```python
from build123d import *

# Parameters (mm, degrees)
FILLET1_SIZE              = 1.27
FILLET1_SIZE_2            = 12.7
SKETCH3_W                 = 3.175
SKETCH3_H                 = 3.175
CUT_EXTRUDE1_DEPTH        = 46.228
F_4_40_TAPPED_HOLE1_D     = 2.2606
F_4_40_TAPPED_HOLE1_DEPTH = 7.62
F_4_40_TAPPED_HOLE1_TIP   = 0.679152758
CIRPATTERN1_COUNT         = 4
BOSS_EXTRUDE1_DEPTH       = 41.402


# Read off the part's stored shape, not the designer's step: #6-32 Tapped Hole1
with BuildPart() as part:
    # Sketch2 → Revolve1 (revolve)
    with BuildSketch(Plane.XY, mode=Mode.PRIVATE) as revolve1_sk:
        Polygon((50.8, 0), (-115.824, 0), (-115.824, 4.7625), (-103.124, 4.7625), (-103.124, 38.862), (-10.16, 38.862), (-9.525, 38.227), (-9.525, 38.862), (0, 38.862), (0, 17.4498), (4.572, 17.4498), (4.572, 6.6675), (50.165, 6.6675), (50.8, 6.0325), align=None)
    revolve(revolve1_sk.sketch.rotate(Axis((88.99, 0, 0), (-1, 0, 0)), 90), axis=Axis((88.99, 0, 0), (-1, 0, 0)))

    # Fillet1
    # an asymmetric fillet: 12.7, 1.27 mm, written as the material it takes off along each edge
    with BuildSketch(Plane(origin=(-103.124, 0, 0), x_dir=(0, 0, -1), z_dir=(0, 1, 0))) as fillet1_piece_1:
        with BuildLine():
            Bezier((38.862 - FILLET1_SIZE, 0), (38.862, 0), (38.862, -FILLET1_SIZE_2), weights=[1, 0.707106781, 1])
            Line((38.862, -FILLET1_SIZE_2), (38.862, 0))
            Line((38.862, 0), (38.862 - FILLET1_SIZE, 0))
        make_face()
    revolve(axis=Axis((-103.124, 0, 0), (-1, 0, 0)), mode=Mode.SUBTRACT)

    # Sketch3 → Cut-Extrude1 (cut)
    with BuildSketch(Plane(origin=(50.8, 0, 0), x_dir=(0, 0, -1), z_dir=(1, 0, 0))):
        with Locations((0, 6.6675)):
            Rectangle(SKETCH3_W, SKETCH3_H)
    extrude(amount=-CUT_EXTRUDE1_DEPTH, mode=Mode.SUBTRACT)

    # Sketch8 → #8-32 Tapped Hole3 (revolve, cut)
    with BuildSketch(Plane(origin=(0, 0, -25), x_dir=(0, 0, -1), z_dir=(0, 1, 0))):
        Polygon((0, 0), (0, 11.705806461), (1.7272, 10.668), (1.7272, 0), align=None)
    f_8_32_tapped_hole3 = revolve(axis=Axis((6.35, 0, -25), (-1, 0, 0)), mode=Mode.SUBTRACT)

    # #6-32 Tapped Hole1 outline → #6-32 Tapped Hole1 (revolve, cut)
    with BuildSketch(Plane(origin=(0, 19.813624417, 28.296788218), x_dir=(0, 1, 0), z_dir=(0, 0, -1))):
        Polygon((1.35255, -93.726), (0, -92.91330597), (0, -103.124), (1.35255, -103.124), align=None)
    f_6_32_tapped_hole1 = revolve(axis=Axis((0, 19.813624417, 28.296788218), (1, 0, 0)), mode=Mode.SUBTRACT)

    # #4-40 Tapped Hole1
    with Locations(Plane.ZY.offset(103.124)):
        with Locations((-23, 0), (23, 0)):
            Hole(F_4_40_TAPPED_HOLE1_D / 2, depth=F_4_40_TAPPED_HOLE1_DEPTH)
            with Locations((0, 0, -(F_4_40_TAPPED_HOLE1_DEPTH + F_4_40_TAPPED_HOLE1_TIP / 2))):  # 118° drill point
                Cone(0, F_4_40_TAPPED_HOLE1_D / 2, F_4_40_TAPPED_HOLE1_TIP, mode=Mode.SUBTRACT)

    # CirPattern1: #8-32 Tapped Hole3, #6-32 Tapped Hole1 ×4 about axis
    cirpattern1_axis = Axis((0, 0, 0), (1, 0, 0))
    add([f_8_32_tapped_hole3.rotate(cirpattern1_axis, i * 360 / CIRPATTERN1_COUNT) for i in range(1, CIRPATTERN1_COUNT)], mode=Mode.SUBTRACT)
    add([f_6_32_tapped_hole1.rotate(cirpattern1_axis, i * 360 / CIRPATTERN1_COUNT) for i in range(1, CIRPATTERN1_COUNT)], mode=Mode.SUBTRACT)

    # Sketch12 → Boss-Extrude1 (add)
    with BuildSketch(Plane(origin=(0, 0, 0), x_dir=(1, 0, 0), z_dir=(0, 1, 0))):
        with BuildLine():
            Line((-92.964, -5.08), (-82.804, -5.08))
            ThreePointArc((-82.804, -5.08), (-77.724, 0), (-82.804, 5.08))
            Line((-82.804, 5.08), (-92.964, 5.08))
            Line((-92.964, 5.08), (-92.964, -5.08))
        make_face()
    extrude(amount=BOSS_EXTRUDE1_DEPTH)


solid = part.part
```
The model under review builds one solid part; all positions refer to its coordinate system, in mm. A direction names the side the tool comes from. Give positions to 0.01 mm unless a question says otherwise; leave off trailing zeros. Write each loop counter-clockwise with the first axis right and the second up, starting at its lowest first coordinate (ties: lowest second). Pieces come first, ordered by that corner, then holes.
(1) The part is to be moulded in two halves that separate along Y. For faces 4 (the cylindrical face through (27.688, -6.662, -0.271)), 5 (the flat face through (-115.824, 0, 0)), 6 (the conical face through (-11.526, -24.779, 0.203)), say which applies: released by +Y, released by -Y, zero draft, split by the parting line, or undercut.
(2) Consider section B-B, the plane x = -37. Give the boundary of the cut face in (y, z), and give its area (3 significant figures).
(3) For P1, Ø5.5, axis at y = 0, z = 25, coming from the +X side; P2, Ø12, axis at x = -44.5, y = 28, coming from the -Z side; P3, Ø3, axis at y = -25, z = 0, coming from the +X side, all flat-tipped, find the tip position at first contact; note any pin that passes through.
(4) Consider section C-C, the plane x = -88. Give the boundary of the cut face in (y, z).
(5) To check wall thickness, follow L1, parallel to X at y = -5.5, z = -9; L2, parallel to Z at x = -97.25, y = 0; L3, parallel to X at y = 31, z = 14. State the ranges of each line that lie inside material, in increasing order.
(6) Consider section A-A, the plane x = 28. Give the boundary of the cut face in (y, z) (1 decimal).
(7) Tool access review of faces 1 (the cylindrical face through (-109.39, 4.65, 1.03)), 2 (the cylindrical face through (-5.259, -23.274, 0.076)), 3 (the cylindrical face through (-77.725, 39.945, 0.112)): name each direction out of +Z, -Z, +X, -X, +Y, -Y from which nothing blocks a thin tool from reaching the whole face with its end or side.
Returned:
1. face 4: split by the parting line
1. face 5: zero draft
1. face 6: undercut
2. outline: circle Ø77.72 at (0, 0)
2. area: 4,740 mm2
3. P1: stops at x = 0
3. P2: stops at z = -32.04
3. P3: stops at x = -10.8
4. outline: (38.53, -5.08) - (41.4, -5.08) - (41.4, 5.08) - (38.53, 5.08) arc R38.86 ccw (long way) to start
5. L1: x = -103.12 to 4.57
5. L2: z = -38.66 to -24.13, -21.87 to 21.87, 24.13 to 38.66
5. L3: x = -103.12 to 0
6. outline: (5.1, -1.6) - (5.1, 1.6) - (6.5, 1.6) arc R6.7 ccw (long way) to (6.5, -1.6) - close
7. face 1: -X
7. face 2: +X
7. face 3: +X, +Y
